Source: CAD feature listing. Evaluate the final solid. Frame: model axes, mm. A direction names the side the tool comes from. Coordinates: 2 decimals unless noted, no trailing zeros. Order: outer loops, then holes, each group sorted by start corner. A loop starts at its lowest first (then second) coordinate and runs counter-clockwise, first axis right, second up.
```python
from build123d import *

# Parameters (mm, degrees)
BOSS_EXTRUDE1_DEPTH = 50
BOSS_EXTRUDE2_DEPTH = 100
SKETCH4_R           = 20
BOSS_EXTRUDE3_DEPTH = 40


with BuildPart() as part:
    # Sketch2 → Boss-Extrude1 (new body)
    with BuildSketch(Plane(origin=(0, 0, 0), x_dir=(0, 0, -1), z_dir=(1, 0, 0))):
        with BuildLine():
            Line((-20, 40), (-20, -40))
            ThreePointArc((-20, -40), (0, -60), (20, -40))
            Line((20, -40), (20, 40))
            ThreePointArc((20, 40), (0, 60), (-20, 40))
        make_face()
        with BuildLine():
            Line((-12.5, 40), (-12.5, -40))
            ThreePointArc((-12.5, -40), (0, -52.5), (12.5, -40))
            Line((12.5, -40), (12.5, 40))
            ThreePointArc((12.5, 40), (0, 52.5), (-12.5, 40))
        make_face(mode=Mode.SUBTRACT)
    extrude(amount=-BOSS_EXTRUDE1_DEPTH)

    # Sketch3 → Boss-Extrude2 (add)
    with BuildSketch(Plane.XY.offset(20)):
        Polygon((-50, 40), (-10, 40), (-10, -40), (-50, -40), (-50, -18), (-38, -18), (-38, -24.542301432), (-22, -24.542301432), (-22, 31.457698568), (-38, 31.457698568), (-38, 18), (-50, 18), align=None)
    extrude(amount=BOSS_EXTRUDE2_DEPTH)

    # Sketch4 → Boss-Extrude3 (add)
    with BuildSketch(Plane(origin=(0, 40, 0), x_dir=(1, 0, 0), z_dir=(0, 1, 0))):
        with Locations(Location((-30, -70, 0), (0, 0, 180))):
            Circle(SKETCH4_R)
    extrude(amount=BOSS_EXTRUDE3_DEPTH)


solid = part.part
```
1. Pin query (flat end, axial travel): P1, Ø2, axis at x = -29.5, z = 25, coming from the +Y side; P2, Ø12, axis at x = -33.5, z = 19, coming from the +Y side; P3, Ø17, axis at y = 2, z = 92, coming from the -X side. Return the tip coordinate at first contact, or that it passes through.
Findings:
P1: stops at y = 40
P2: stops at y = 55.2
P3: stops at x = -22
2. Ray query, line 1 (Z direction, x = -13, y = -14); line 2 (Z direction, x = -41, y = 48); line 3 (Y direction, x = -33, z = 78). Return the intervals inside material, ascending.
Findings:
line 1: z = -20 to -12.5, 12.5 to 120
line 2: z = -18.33 to -9.6, 9.6 to 18.33, 53.3 to 86.7
line 3: y = -40 to -24.54, 31.46 to 80
3. Section query C-C on y = 48. Return loops of the section in (x, z), plus the area to 3 significant figures.
Findings:
outline: (-50, -18.33) - (0, -18.33) - (0, -9.6) - (-50, -9.6) - close; (-50, 9.6) - (0, 9.6) - (0, 18.33) - (-50, 18.33) - close; circle Ø40 at (-30, 70)
area: 2,130 mm2
4. Section query D-D on x = -30. Return loops of the section in (y, z).
Findings:
outline: (-40, -20) - (40, -20) arc R20 ccw to (40, 20) - (40, 50) - (80, 50) - (80, 90) - (40, 90) - (40, 120) - (31.46, 120) - (31.46, 20) - (-24.54, 20) - (-24.54, 120) - (-40, 120) - (-40, 20) arc R20 ccw to start; hole (-40, -12.5) - (40, -12.5) arc R12.5 ccw to (40, 12.5) - (-40, 12.5) arc R12.5 ccw to start
5. Section query A-A on x = -7.5. Return loops of the section in (y, z).
Findings:
outline: (-40, -20) - (40, -20) arc R20 ccw to (40, 20) - (-40, 20) arc R20 ccw to start; hole (-40, -12.5) - (40, -12.5) arc R12.5 ccw to (40, 12.5) - (-40, 12.5) arc R12.5 ccw to start
6. Access query for faces 4 (the face through (-38, 25, 69)), 5 (the face through (-25, -1, -12.5)), 6 (the face through (-44, 18, 69)). Directions: +Z, -Z, +X, -X, +Y, -Y. A direction counts if a zero-diameter tool reaches every point of the face in a straight line with its end or side. Return the directions, or none.
Findings:
face 4: +Z
face 5: +X, -X
face 6: +Z, -X
7. Section query B-B on z = 0. Return loops of the section in (x, y).
Findings:
outline: (-50, -60) - (0, -60) - (0, -52.5) - (-50, -52.5) - close; (-50, 52.5) - (0, 52.5) - (0, 60) - (-50, 60) - close
8. Draft query along Y for faces 1 (the face through (-25, 60, 0)), 2 (the face through (-25, 1, 12.5)), 3 (the face through (-25, -1, -20)). Return one class per face: released by +Y, released by -Y, zero draft, split by the parting line, or undercut.
Findings:
face 1: released by +Y
face 2: undercut
face 3: zero draft
